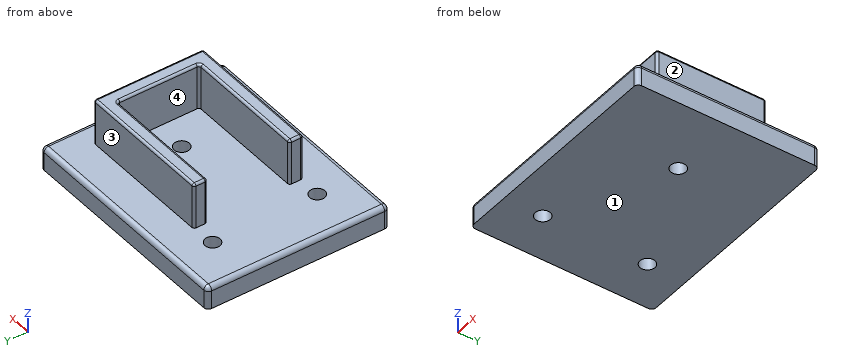
from build123d import *

# Parameters (mm, degrees)
SKETCH_2_W          = 50
SKETCH_2_H          = 40
EXTRUDE_1_DEPTH     = 5
EXTRUDE_START       = -8
SKETCH_5_W          = 30
SKETCH_5_H          = 10
EXTRUDE_2_DEPTH     = 3
SKETCH_6_W          = 30
SKETCH_6_H          = 10
EXTRUDE_3_DEPTH     = 3
CUT_EXTRUDE_1_REACH = 86.906
SKETCH_7_R          = 1.65
FILLET_3_R          = 1
SKETCH_8_W          = 10
SKETCH_8_H          = 21
EXTRUDE_4_DEPTH     = 3
FILLET_4_R          = 0.5


with BuildPart() as part:
    # 草图2 → 凸台-拉伸1 (new body)
    with BuildSketch(Plane.XY):
        with Locations((53, 10)):
            Rectangle(SKETCH_2_W, SKETCH_2_H)
    extrude(amount=EXTRUDE_1_DEPTH)

    # 草图5 → 凸台-拉伸2 (add)
    with BuildSketch(Plane.XZ.offset(10).offset(EXTRUDE_START)):
        with Locations((58, 10)):
            Rectangle(SKETCH_5_W, SKETCH_5_H)
    extrude(amount=-EXTRUDE_2_DEPTH)

    # 草图6 → 凸台-拉伸3 (add)
    with BuildSketch(Plane(origin=(0, 30, 0), x_dir=(1, 0, 0), z_dir=(0, 1, 0)).offset(EXTRUDE_START)):
        with Locations((58, -10)):
            Rectangle(SKETCH_6_W, SKETCH_6_H)
    extrude(amount=-EXTRUDE_3_DEPTH)

    # 草图7 → 切除-拉伸1 (cut, up to next)
    with BuildSketch(Plane(origin=(0, 0, 0), x_dir=(-1, 0, 0), z_dir=(0, 0, -1)), mode=Mode.PRIVATE) as cut_extrude_1_sk1:
        with Locations((-63, 10)):
            Circle(SKETCH_7_R)
    cut_extrude_1_tool1 = extrude(cut_extrude_1_sk1.sketch, amount=-CUT_EXTRUDE_1_REACH, mode=Mode.PRIVATE) & part.part
    # 草图7 → 切除-拉伸1 (cut, up to next)
    with BuildSketch(Plane(origin=(0, 0, 0), x_dir=(-1, 0, 0), z_dir=(0, 0, -1)), mode=Mode.PRIVATE) as cut_extrude_1_sk2:
        with Locations((-38, -1.5)):
            Circle(SKETCH_7_R)
    cut_extrude_1_tool2 = extrude(cut_extrude_1_sk2.sketch, amount=-CUT_EXTRUDE_1_REACH, mode=Mode.PRIVATE) & part.part
    # 草图7 → 切除-拉伸1 (cut, up to next)
    with BuildSketch(Plane(origin=(0, 0, 0), x_dir=(-1, 0, 0), z_dir=(0, 0, -1)), mode=Mode.PRIVATE) as cut_extrude_1_sk3:
        with Locations((-38, 21.5)):
            Circle(SKETCH_7_R)
    cut_extrude_1_tool3 = extrude(cut_extrude_1_sk3.sketch, amount=-CUT_EXTRUDE_1_REACH, mode=Mode.PRIVATE) & part.part
    add(cut_extrude_1_tool1.solids().sort_by_distance((63, 10, 0))[0], mode=Mode.SUBTRACT)
    add(cut_extrude_1_tool2.solids().sort_by_distance((38, -1.5, 0))[0], mode=Mode.SUBTRACT)
    add(cut_extrude_1_tool3.solids().sort_by_distance((38, 21.5, 0))[0], mode=Mode.SUBTRACT)

    # 圆角3
    fillet_3_edges = [part.edges().sort_by_distance(p)[0] for p in [
        (28, 10, 5),
        (53, -10, 5),
        (78, 10, 5),
        (78, -10, 2.5),
        (28, -10, 2.5),
        (28, 30, 2.5),
        (78, 30, 2.5),
        (53, 30, 5),
    ]]
    fillet(fillet_3_edges, radius=FILLET_3_R)

    # 草图8 → 凸台-拉伸4 (add)
    with BuildSketch(Plane(origin=(73, 0, 0), x_dir=(0, 0, -1), z_dir=(1, 0, 0))):
        with Locations((-10, 8.5)):
            Rectangle(SKETCH_8_W, SKETCH_8_H)
    extrude(amount=-EXTRUDE_4_DEPTH)

    # 圆角4
    fillet_4_edges = [part.edges().sort_by_distance(p)[0] for p in [
        (43, 1, 10),
        (43, -0.5, 15),
        (73, 10, 15),
        (73, -2, 10),
        (58, -2, 15),
        (43, -2, 10),
        (56.5, 19, 15),
        (43, 19, 10),
        (43, 20.5, 15),
        (43, 22, 10),
        (58, 22, 15),
        (73, 22, 10),
        (56.5, 1, 15),
        (70, 10, 15),
        (70, 1, 10),
        (70, 19, 10),
    ]]
    fillet(fillet_4_edges, radius=FILLET_4_R)


solid = part.part
Here's how the part is built. I have some questions about the finished solid (model axes, mm). Face numbers are marked on the shaded views. A direction names the side the tool comes from. Coordinates: 2 decimals unless noted, no trailing zeros. Write each loop counter-clockwise with the first axis right and the second up, starting at its lowest first coordinate (ties: lowest second). Pieces come first, ordered by that corner, then holes.
1) If I drill on line 1 (Y direction, x = 38, z = 3.4); line 2 (Z direction, x = 74.5, y = -3.5); line 3 (X direction, y = 4.5, z = 5.5), over which ranges is the centre line in solid material (lowest first)?
Filled in:
line 1: y = -10 to -3.15, 0.15 to 19.85, 23.15 to 30
line 2: z = 0 to 5
line 3: x = 70 to 73
2) If we section it at D-D (y = 10): List the corners of the cut face in (x, z) for me, plus the area to 3 significant figures.
Filled in:
outline: (28, 0) - (61.35, 0) - (61.35, 5) - (29, 5) arc R1 ccw to (28, 4) - close; (64.65, 0) - (78, 0) - (78, 4) arc R1 ccw to (77, 5) - (73, 5) - (73, 14.5) arc R0.5 ccw to (72.5, 15) - (70.5, 15) arc R0.5 ccw to (70, 14.5) - (70, 5) - (64.65, 5) - close
area: 263 mm2
3) If we section it at B-B (x = 63): List the corners of the cut face in (y, z) for me, plus the area to 3 significant figures.
Filled in:
outline: (-10, 0) - (8.35, 0) - (8.35, 5) - (1, 5) - (1, 14.5) arc R0.5 ccw to (0.5, 15) - (-1.5, 15) arc R0.5 ccw to (-2, 14.5) - (-2, 5) - (-9, 5) arc R1 ccw to (-10, 4) - close; (11.65, 0) - (30, 0) - (30, 4) arc R1 ccw to (29, 5) - (22, 5) - (22, 14.5) arc R0.5 ccw to (21.5, 15) - (19.5, 15) arc R0.5 ccw to (19, 14.5) - (19, 5) - (11.65, 5) - close
area: 243 mm2
4) If we section it at A-A (x = 38): List the corners of the cut face in (y, z) for me, plus the area to 3 significant figures.
Filled in:
outline: (-10, 0) - (-3.15, 0) - (-3.15, 5) - (-9, 5) arc R1 ccw to (-10, 4) - close; (0.15, 0) - (19.85, 0) - (19.85, 5) - (0.15, 5) - close; (23.15, 0) - (30, 0) - (30, 4) arc R1 ccw to (29, 5) - (23.15, 5) - close
area: 167 mm2
5) Which directions (+Z, -Z, +X, -X, +Y, -Y) give clear straight access to the entire face, cutting with the end or side of a thin tool? Please do the marked faces 1, 2, 3 and 4.
Filled in:
face 1: -Z, +X, -X, +Y, -Y
face 2: +Z, +X, +Y, -Y
face 3: +Z, +X, -X, +Y
face 4: +Z, -X
6) If we section it at C-C (z = 8): List the corners of the cut face in (x, y) for me.
Filled in:
outline: (43, -1.5) arc R0.5 ccw to (43.5, -2) - (72.5, -2) arc R0.5 ccw to (73, -1.5) - (73, 21.5) arc R0.5 ccw to (72.5, 22) - (43.5, 22) arc R0.5 ccw to (43, 21.5) - (43, 19.5) arc R0.5 ccw to (43.5, 19) - (69.5, 19) arc R0.5 cw to (70, 18.5) - (70, 1.5) arc R0.5 cw to (69.5, 1) - (43.5, 1) arc R0.5 ccw to (43, 0.5) - close
7) I'm going to push flat-ended pins straight in: pin 1 (7.5 mm diameter, centred on x = 55.5, z = 10.5, fed in from -Y); pin 2 (1.6 mm diameter, centred on y = -1, z = 9.5, fed in from -X); pin 3 (7.5 mm diameter, centred on y = 9.5, z = 8.5, fed in from +X). Where does each tip first touch, or does it pass through?
Filled in:
pin 1: stops at y = -2
pin 2: stops at x = 43
pin 3: stops at x = 77.66
